Source: CAD feature listing. Evaluate the final solid. Frame: model axes, mm. A direction names the side the tool comes from. Round coordinates to 2 decimals unless told otherwise and drop trailing zeros. Loops run counter-clockwise (first coordinate to the right, second up) from the corner with the lowest first, then second, coordinate; pieces in that order, holes last. Notation, with made-up numbers: M 75,-3 L 106,-3 A26 cw 106,25 Z; hole C 17.5,64 d10. An arc over 180 degrees is marked long. Write each question's results on one line, items separated by ' | '. Start each with the question number.
1. Ray query, line 1 (X direction, y = 2.25, z = 48.5); line 2 (Z direction, x = 1, y = 10.25); line 3 (X direction, y = 1.25, z = 66). Return the intervals inside material, ascending.
2. Section B-B on y = 8. Output: boundary loops of the cut face in (x, z), and give its area (3 significant figures).
3. Set-up query: faces 1 (the flat face through (-78, 6, 0)), 2 (the cylindrical face through (-70.77, 6.26, 64.12)). Return all of +Z, -Z, +X, -X, +Y, -Y with unobstructed straight access to the full face (end or side cutting, diameter ignored); none if empty.
4. Draft query along X for faces 3 (the flat face through (76.2, 6, 26)), 4 (the flat face through (-1, 6, 69.85)), 5 (the flat face through (-80.264, 6, 26)), 6 (the flat face through (1, 6, 73.914)). Return one class per face: released by +X, released by -X, zero draft, split by the parting line, or undercut.
5. Section A-A on z = 49. Output: boundary loops of the cut face in (x, y).
6. Section D-D on x = 42. Output: boundary loops of the cut face in (y, z).
7. Section C-C on z = 65. Output: boundary loops of the cut face in (x, y).
from build123d import *

# Parameters (mm, degrees)
BOSS_EXTRUDE4_DEPTH = 12.7


with BuildPart() as part:
    # Sketch474 → Boss-Extrude4 (new body)
    with BuildSketch(Plane(origin=(0, 0, 0), x_dir=(1, 0, 0), z_dir=(0, 1, 0))):
        with BuildLine():
            Line((-76.2, 0), (-76.2, -50.8))
            ThreePointArc((-76.2, -50.8), (-70.620384182, -64.270384182), (-57.15, -69.85))
            Line((-57.15, -69.85), (57.15, -69.85))
            ThreePointArc((57.15, -69.85), (70.620384182, -64.270384182), (76.2, -50.8))
            Line((76.2, -50.8), (76.2, 0))
            Line((76.2, 0), (80.264, 0))
            Line((80.264, 0), (80.264, -50.8))
            ThreePointArc((80.264, -50.8), (73.49406614, -67.14406614), (57.15, -73.914))
            Line((57.15, -73.914), (-57.15, -73.914))
            ThreePointArc((-57.15, -73.914), (-73.49406614, -67.14406614), (-80.264, -50.8))
            Line((-80.264, -50.8), (-80.264, 0))
            Line((-80.264, 0), (-76.2, 0))
        make_face()
    extrude(amount=BOSS_EXTRUDE4_DEPTH)


solid = part.part
Taken from the geometry:
1) line 1: -80.26 to -76.2, 76.2 to 80.26 | line 2: 69.85 to 73.91 | line 3: -74.56 to -68.63, 68.63 to 74.56
2) outline: M -80.26,0 L -76.2,0 L -76.2,50.8 A19.05 cw -57.15,69.85 L 57.15,69.85 A19.05 cw 76.2,50.8 L 76.2,0 L 80.26,0 L 80.26,50.8 A23.11 ccw 57.15,73.91 L -57.15,73.91 A23.11 ccw -80.26,50.8 Z | area: 1,150 mm^2
3) face 1: -Z, +X, -X, +Y, -Y | face 2: -Z, +Y, -Y
4) face 3: undercut | face 4: undercut | face 5: released by -X | face 6: zero draft
5) outline: M -80.26,0 L -76.2,0 L -76.2,12.7 L -80.26,12.7 Z; M 76.2,0 L 80.26,0 L 80.26,12.7 L 76.2,12.7 Z
6) outline: M 0,69.85 L 12.7,69.85 L 12.7,73.91 L 0,73.91 Z
7) outline: M -75.39,0 L -69.85,0 L -69.85,12.7 L -75.39,12.7 Z; M 69.85,0 L 75.39,0 L 75.39,12.7 L 69.85,12.7 Z
